Geometry: see drawing. Coordinates: mm, zero at the bounding-box minimum. A direction names the side the tool comes from. Coordinates: 2 decimals unless noted, no trailing zeros. Order: outer loops, then holes, each group sorted by start corner. A loop starts at its lowest first (then second) coordinate and runs counter-clockwise, first axis right, second up.
Item 1: Contact query for flat-ended pins moving along their axis: P1, Ø5, axis at x = 77, z = 13.5, coming from the -Y side; P2, Ø4, axis at y = 28.5, z = 22.5, coming from the -X side; P3, Ø5, axis at x = 39, y = 30, coming from the +Z side. Output: stop coordinate, or through.
Item 2: Section D-D on y = 39. Return the cut outline in (x, z) (1 decimal).
Item 3: Ray query, line 1 (Z direction, x = 68.5, y = 42) (1 decimal); line 2 (Y direction, x = 64.5, z = 3); line 3 (Z direction, x = 24.5, y = 41). Return the intervals inside material, ascending.
Item 4: Mould query, pull axis X, two halves, no side actions, for the marked faces 4, 5 and 6. Classes: released by +X, released by -X, zero draft, split by the parting line, or undercut.
Item 5: Section C-C on z = 18.5. Return the cut outline in (x, y) (1 decimal).
Item 6: Section B-B on x = 63.5. Return the cut outline in (y, z).
Item 7: Section A-A on y = 16. Return the cut outline in (x, z) (1 decimal).
Item 8: Reachability of the marked faces 1, 2 and 3 from +Z, -Z, +X, -X, +Y, -Y: full face, straight path, thin tool, end or side. Return the list, or none.
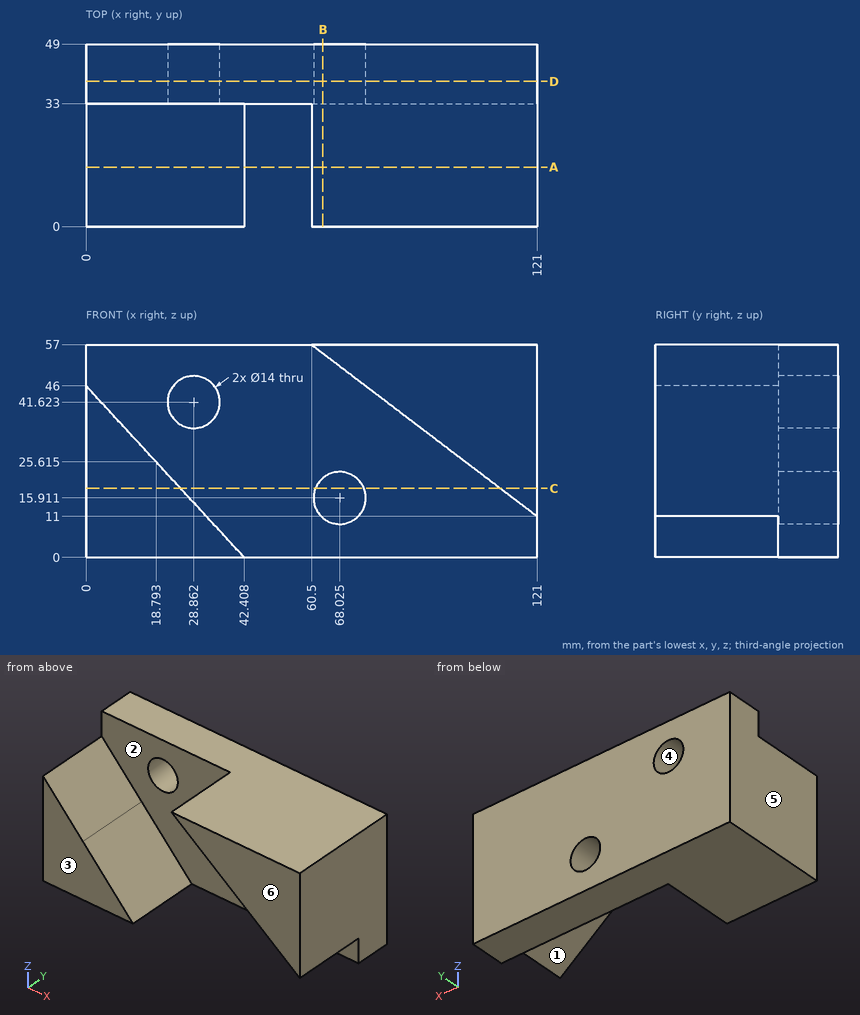
Answer list:
1. P1: stops at y = 33
1. P2: stops at x = 0
1. P3: stops at z = 6.41
2. outline: (0, 0) - (121, 0) - (121, 57) - (0, 57) - close; hole circle Ø14 at (28.9, 41.6); hole circle Ø14 at (68, 15.9)
3. line 1: z = 0 to 8.9, 22.9 to 57
3. line 2: y = 33 to 49
3. line 3: z = 0 to 36.15, 47.1 to 57
4. face 4: undercut
4. face 5: released by -X
4. face 6: zero draft
5. outline: (0, 0) - (25.4, 0) - (25.4, 33) - (61.5, 33) - (61.5, 49) - (0, 49) - close; (74.5, 33) - (111.1, 33) - (111.1, 0) - (121, 0) - (121, 49) - (74.5, 49) - close
6. outline: (0, 54.72) - (33, 54.72) - (33, 21.25) - (49, 21.25) - (49, 57) - (0, 57) - close; (33, 0) - (49, 0) - (49, 10.57) - (33, 10.57) - close
7. outline: (0, 0) - (42.4, 0) - (0, 46) - close; (60.5, 57) - (121, 11) - (121, 57) - close
8. face 1: -Z, -Y
8. face 2: -Y
8. face 3: +Z, -Z, +X, -X, -Y
